Drawing for the job (mm, zero at the part's lowest x, y, z). Round coordinates to 2 decimals unless told otherwise and drop trailing zeros. Loops run counter-clockwise (first coordinate to the right, second up) from the corner with the lowest first, then second, coordinate; pieces in that order, holes last. Notation, with made-up numbers: M 81,6.25 L 132,6.25 A13 ccw 132,22.25 Z; hole C 30,43.5 d11. An arc over 180 degrees is marked long. Use a Markdown table: item, result. Add a question column.
Q1. Cut at B-B (x = 22.9). Give the cut face in (y, z) (3 decimals), plus the area to 3 significant figures.
Q2. Cut at C-C (z = 2.95). State how many separate pieces and enclosed holes the cut face has, plus the area to 3 significant figures.
Q3. Pin check, flat tips, straight feed: pin 1 (2 mm diameter, centred on y = 37, z = 2, fed in from -X); pin 2 (3 mm diameter, centred on x = 27.5, y = 57, fed in from -Z). Stop position of each tip, or through.
Q4. Cut at D-D (x = 32). Give the cut face in (y, z) (3 decimals).
Q5. Cut at A-A (y = 31.5). Give the cut face in (x, z), plus the area to 3 significant figures.
Q6. Probe line 1 (X direction, y = 36, z = 2.5); line 2 (Y direction, x = 32.9, z = 0.95) (3 decimals); line 3 (X direction, y = 60.5, z = 0.7). List the from-to ranges inside material, lowest first. Write a range as from..to.
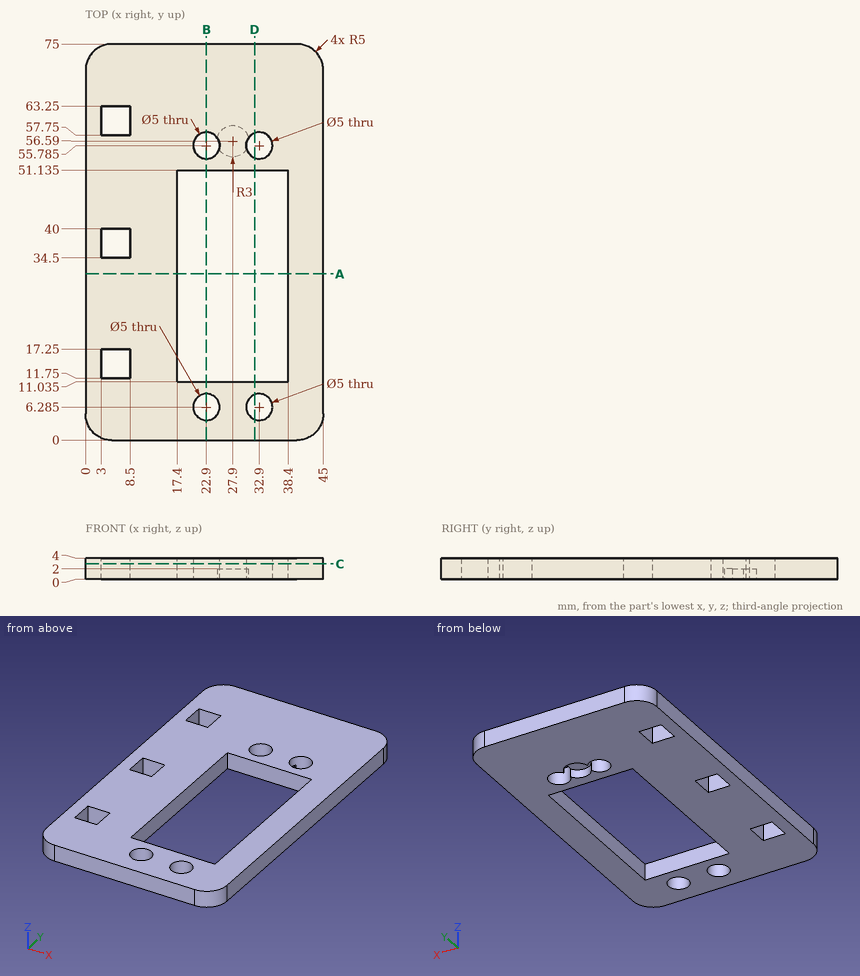
Checked values:
| question | item | result |
|---|---|---|
| 1 | outline | M 0,0 L 3.785,0 L 3.785,4 L 0,4 Z; M 8.785,0 L 11.035,0 L 11.035,4 L 8.785,4 Z; M 51.135,0 L 53.285,0 L 53.285,4 L 51.135,4 Z; M 58.285,0 L 75,0 L 75,4 L 58.285,4 Z |
| 1 | area | 99.6 mm^2 |
| 2 | separate pieces | 1 |
| 2 | enclosed holes | 8 |
| 2 | area | 2,340 mm^2 |
| 3 | pin 1 | stops at x = 0 |
| 3 | pin 2 | stops at z = 2 |
| 4 | outline | M 0,0 L 3.953,0 L 3.953,4 L 0,4 Z; M 8.617,0 L 11.035,0 L 11.035,4 L 8.617,4 Z; M 51.135,0 L 53.453,0 L 53.453,4 L 51.135,4 Z; M 58.117,0 L 75,0 L 75,4 L 58.117,4 Z |
| 5 | outline | M 0,0 L 17.4,0 L 17.4,4 L 0,4 Z; M 38.4,0 L 45,0 L 45,4 L 38.4,4 Z |
| 5 | area | 96.0 mm^2 |
| 6 | line 1 | x = 0..3, 8.5..17.4, 38.4..45 |
| 6 | line 2 | y = 0..3.785, 8.785..11.035, 51.135..53.285, 58.285..75 |
| 6 | line 3 | x = 0..3, 8.5..45 |
